Autodesk Inventor part; units mm, degrees
ref_plane "YZ Plane" through (0, 0, 0) normal (1, 0, 0) x (0, 1, 0)
ref_plane "XZ Plane" through (0, 0, 0) normal (0, 1, 0) x (-1, 0, 0)
ref_plane "XY Plane" through (0, 0, 0) normal (0, 0, 1) x (1, 0, 0)
sketch "Sketch1" plane through (0, 0, 0) normal (0, 0, 1) x (1, 0, 0)
  line L0 (-12.7, 12.7) -> (12.7, 12.7)
  line L1 (12.7, 12.7) -> (12.7, -12.7)
  line L2 (12.7, -12.7) -> (-12.7, -12.7)
  line L3 (-12.7, -12.7) -> (-12.7, 12.7)
  point P0 (0, 0)
  dimension "d0" = 25.4
  dimension "d1" = 25.4
  dimension "d2" = 12.7
  dimension "d3" = 12.7
extrude "Extrusion1" add sketch "Sketch1" along normal blind 50.8
sketch "Sketch2" plane through (0, 0, 50.8) normal (0, 0, 1) x (1, 0, 0)
  circle A0 centre (0, 0) radius 2.54
  line L0 (-4.5085, 4.5085) -> (4.5085, 4.5085)
  line L1 (-4.5085, -4.5085) -> (4.5085, -4.5085)
  line L2 (4.5085, 4.5085) -> (4.5085, -4.5085)
  line L3 (-4.5085, 4.5085) -> (-4.5085, -4.5085)
  line L4 (-3.0896, 4.5085) -> (-11.2811, 12.7)
  line L5 (-4.5085, 3.0537) -> (-12.7, 11.2452)
  line L6 (12.7, 12.7) -> (-12.7, 12.7)
  line L7 (-12.7, 12.7) -> (-12.7, 4.0005)
  line L8 (-10.668, 4.0005) -> (-10.668, 9.2132)
  line L9 (-9.2491, 10.668) -> (-3.3655, 10.668)
  line L10 (-12.7, 12.7) -> (-3.3655, 12.7)
  line L11 (-2.7305, 11.303) -> (-2.7305, 12.065)
  line L12 (-12.065, 3.3655) -> (-11.303, 3.3655)
  arc A1 (-12.7, 4.0005) -> (-12.065, 3.3655) centre (-12.065, 4.0005) ccw
  arc A2 (-11.303, 3.3655) -> (-10.668, 4.0005) centre (-11.303, 4.0005) ccw
  arc A3 (-3.3655, 10.668) -> (-2.7305, 11.303) centre (-3.3655, 11.303) ccw
  arc A4 (-2.7305, 12.065) -> (-3.3655, 12.7) centre (-3.3655, 12.065) ccw
  arc A5 (-3.3655, -11.303) -> (-4.0005, -10.668) centre (-4.0005, -11.303) ccw
  line L13 (-3.3655, -12.065) -> (-3.3655, -11.303)
  arc A6 (-4.0005, -12.7) -> (-3.3655, -12.065) centre (-4.0005, -12.065) ccw
  line L14 (-3.0537, -4.5085) -> (-11.2452, -12.7)
  line L15 (-10.668, -9.2491) -> (-10.668, -3.3655)
  line L16 (-4.5085, -3.0896) -> (-12.7, -11.2811)
  line L17 (-12.7, -12.7) -> (-12.7, -3.3655)
  arc A7 (-10.668, -3.3655) -> (-11.303, -2.7305) centre (-11.303, -3.3655) ccw
  line L18 (-11.303, -2.7305) -> (-12.065, -2.7305)
  arc A8 (-12.065, -2.7305) -> (-12.7, -3.3655) centre (-12.065, -3.3655) ccw
  line L19 (-4.0005, -10.668) -> (-9.2132, -10.668)
  line L20 (-12.7, -12.7) -> (-4.0005, -12.7)
  arc A9 (11.303, -3.3655) -> (10.668, -4.0005) centre (11.303, -4.0005) ccw
  line L21 (12.065, -3.3655) -> (11.303, -3.3655)
  arc A10 (12.7, -4.0005) -> (12.065, -3.3655) centre (12.065, -4.0005) ccw
  line L22 (4.5085, -3.0537) -> (12.7, -11.2452)
  line L23 (9.2491, -10.668) -> (3.3655, -10.668)
  line L24 (3.0896, -4.5085) -> (11.2811, -12.7)
  line L25 (12.7, -12.7) -> (3.3655, -12.7)
  arc A11 (3.3655, -10.668) -> (2.7305, -11.303) centre (3.3655, -11.303) ccw
  line L26 (2.7305, -11.303) -> (2.7305, -12.065)
  arc A12 (2.7305, -12.065) -> (3.3655, -12.7) centre (3.3655, -12.065) ccw
  line L27 (10.668, -4.0005) -> (10.668, -9.2132)
  line L28 (12.7, -12.7) -> (12.7, -4.0005)
  arc A13 (3.3655, 11.303) -> (4.0005, 10.668) centre (4.0005, 11.303) ccw
  line L29 (3.3655, 12.065) -> (3.3655, 11.303)
  arc A14 (4.0005, 12.7) -> (3.3655, 12.065) centre (4.0005, 12.065) ccw
  line L30 (3.0537, 4.5085) -> (11.2452, 12.7)
  line L31 (10.668, 9.2491) -> (10.668, 3.3655)
  line L32 (4.5085, 3.0896) -> (12.7, 11.2811)
  line L33 (12.7, 12.7) -> (12.7, 3.3655)
  arc A15 (10.668, 3.3655) -> (11.303, 2.7305) centre (11.303, 3.3655) ccw
  line L34 (11.303, 2.7305) -> (12.065, 2.7305)
  arc A16 (12.065, 2.7305) -> (12.7, 3.3655) centre (12.065, 3.3655) ccw
  line L35 (4.0005, 10.668) -> (9.2132, 10.668)
  line L36 (12.7, 12.7) -> (4.0005, 12.7)
  line L37 (-4.5085, 3.0537) -> (-4.5085, 4.5085)
  line L38 (-3.0896, 4.5085) -> (-4.5085, 4.5085)
  line L39 (-12.7, -12.7) -> (-4.0005, -12.7)
  line L40 (-4.0005, -10.668) -> (-9.2132, -10.668)
  line L41 (-10.668, -9.2491) -> (-10.668, -3.3655)
  line L42 (-12.7, -12.7) -> (-12.7, -3.3655)
  line L43 (-11.303, -2.7305) -> (-12.065, -2.7305)
  arc A17 (-10.668, -3.3655) -> (-11.303, -2.7305) centre (-11.303, -3.3655) ccw
  arc A18 (-12.065, -2.7305) -> (-12.7, -3.3655) centre (-12.065, -3.3655) ccw
  line L44 (-4.5085, -3.0896) -> (-4.5085, -4.5085)
  line L45 (-4.5085, -3.0896) -> (-12.7, -11.2811)
  line L46 (-3.0537, -4.5085) -> (-4.5085, -4.5085)
  line L47 (-3.0537, -4.5085) -> (-11.2452, -12.7)
  line L48 (-4.5085, -4.5085) -> (-4.5085, 4.5085)
  circle A19 centre (0, 0) radius 2.54
  line L49 (-4.5085, -4.5085) -> (4.5085, -4.5085)
  line L50 (-3.3655, -12.065) -> (-3.3655, -11.303)
  arc A20 (-4.0005, -12.7) -> (-3.3655, -12.065) centre (-4.0005, -12.065) ccw
  arc A21 (-3.3655, -11.303) -> (-4.0005, -10.668) centre (-4.0005, -11.303) ccw
  line L51 (12.7, -12.7) -> (12.7, -4.0005)
  line L52 (10.668, -4.0005) -> (10.668, -9.2132)
  line L53 (9.2491, -10.668) -> (3.3655, -10.668)
  line L54 (12.7, -12.7) -> (3.3655, -12.7)
  line L55 (2.7305, -11.303) -> (2.7305, -12.065)
  arc A22 (3.3655, -10.668) -> (2.7305, -11.303) centre (3.3655, -11.303) ccw
  arc A23 (2.7305, -12.065) -> (3.3655, -12.7) centre (3.3655, -12.065) ccw
  line L56 (3.0896, -4.5085) -> (4.5085, -4.5085)
  line L57 (3.0896, -4.5085) -> (11.2811, -12.7)
  line L58 (4.5085, -3.0537) -> (4.5085, -4.5085)
  line L59 (4.5085, -3.0537) -> (12.7, -11.2452)
  line L60 (4.5085, -4.5085) -> (-4.5085, -4.5085)
  circle A24 centre (0, 0) radius 2.54
  line L61 (4.5085, -4.5085) -> (4.5085, 4.5085)
  line L62 (12.065, -3.3655) -> (11.303, -3.3655)
  arc A25 (12.7, -4.0005) -> (12.065, -3.3655) centre (12.065, -4.0005) ccw
  arc A26 (11.303, -3.3655) -> (10.668, -4.0005) centre (11.303, -4.0005) ccw
  line L63 (12.7, 12.7) -> (4.0005, 12.7)
  line L64 (4.0005, 10.668) -> (9.2132, 10.668)
  line L65 (10.668, 9.2491) -> (10.668, 3.3655)
  line L66 (12.7, 12.7) -> (12.7, 3.3655)
  line L67 (11.303, 2.7305) -> (12.065, 2.7305)
  arc A27 (10.668, 3.3655) -> (11.303, 2.7305) centre (11.303, 3.3655) ccw
  arc A28 (12.065, 2.7305) -> (12.7, 3.3655) centre (12.065, 3.3655) ccw
  line L68 (4.5085, 3.0896) -> (4.5085, 4.5085)
  line L69 (4.5085, 3.0896) -> (12.7, 11.2811)
  line L70 (3.0537, 4.5085) -> (4.5085, 4.5085)
  line L71 (3.0537, 4.5085) -> (11.2452, 12.7)
  line L72 (4.5085, 4.5085) -> (4.5085, -4.5085)
  circle A29 centre (0, 0) radius 2.54
  line L73 (4.5085, 4.5085) -> (-4.5085, 4.5085)
  line L74 (3.3655, 12.065) -> (3.3655, 11.303)
  arc A30 (4.0005, 12.7) -> (3.3655, 12.065) centre (4.0005, 12.065) ccw
  arc A31 (3.3655, 11.303) -> (4.0005, 10.668) centre (4.0005, 11.303) ccw
  point P0 (-12.7, 3.3655)
  point P1 (-2.7305, 12.7)
  point P2 (-3.3655, -12.7)
  point P3 (-12.7, -2.7305)
  point P4 (12.7, -3.3655)
  point P5 (2.7305, -12.7)
  point P6 (3.3655, 12.7)
  point P7 (12.7, 2.7305)
  point P8 (-3.3655, -12.7)
  point P9 (-12.7, -2.7305)
  point P10 (12.7, -3.3655)
  point P11 (2.7305, -12.7)
  point P12 (3.3655, 12.7)
  point P13 (12.7, 2.7305)
  dimension "d6" = 5.08
  dimension "d7" = 9.017
  dimension "d8" = 4.5085
  dimension "d9" = 4.5085
  dimension "d10" = 4.5085
  dimension "d11" = 2.032
  dimension "d12" = 1.0033
  dimension "d13" = 135
  dimension "d17" = 9.3345
  dimension "d19" = 2.032
  dimension "d20" = 2.032
  dimension "d21" = 0.635
  dimension "d22" = 9.3345
  dimension "d25" = 360
  dimension "d29" = 360
extrude "Extrusion2" cut sketch "Sketch2" against normal up to surface (50.8 mm away) contours L3 L5 L7 L6 L4 L0 | L0 L2 L1 L3 | L30 L6 L33 L32 L2 L0 | L4 L6 A4 L11 A3 L9 | L3 L1 L14 L20 L17 L16 | L8 A2 L12 A1 L7 L5 | L35 A13 L29 A14 L6 L30 | L16 L17 A8 L18 A7 L15 | L22 L28 L25 L24 L1 L2 | L32 L33 A16 L34 A15 L31 | L19 A5 L13 A6 L20 L14 | L27 A9 L21 A10 L28 L22 | L24 L25 A12 L26 A11 L23 keep common part
equation "\"d22\" = d17"
properties part number "~2 in 80-20 extrusion"
Check sheet for the modelled part. Datum: model origin and axes. Units: mm. A direction names the side the tool comes from. Give positions to 0.01 mm unless a question says otherwise; leave off trailing zeros. Write each loop counter-clockwise with the first axis right and the second up, starting at its lowest first coordinate (ties: lowest second). Pieces come first, ordered by that corner, then holes. Notation, with made-up numbers: (19.5, -14) -> (74.5, -14) arc R23 ccw to (74.5, 2) -> close; hole circle Ø6 at (-2.75, 45.5). An arc over 180 degrees is marked (long way). Use CSV: the item, a comma, the result in double quotes. Start each with the question number.
Q1. Release check for a two-part mould opening along Y. For faces 3 (the flat face through (7, 10.668, 26)), 4 (the flat face through (0, 3, 0)), 5 (the flat face through (-8, 12.7, 25)) record: +Y half, -Y half, draft (parallel to the pull), parting line (faces both ways), or undercut.
Q2. Cross-section at C-C on y = -5.75. Enter the section's corners in (x, z).
Q3. Scan lines: line 1 along Y through (x, z) = (0, 38); line 2 along Y through (x, z) = (6.5, 10); line 3 along Y through (x, z) = (-5.5, 23). Record each from-to range of solid material in increasing order.
Q4. Cross-section at A-A on y = 0. Enter the section's corners in (x, z).
Q5. Tool access check on faces 1 (the flat face through (-6.09, -7.545, 25.756)), 2 (the flat face through (-8, -12.7, 25)). Record the directions out of +Z, -Z, +X, -X, +Y, -Y that give a thin tool (end or side, any length) a straight path to the whole face; none if there is none.
Q6. Depth check by flat-ended pin: P1, Ø1.5, axis at x = 4.5, y = -9.5, coming from the -Z side; P2, Ø4, axis at y = -3.5, z = 37, coming from the +X side; P3, Ø3, axis at x = 1, z = 30, coming from the -Y side; P4, Ø1.8, axis at y = 1, z = 25.5, coming from the +X side. Enter the tip coordinate at first touch or a pass-through.
Working result:
1,face 3,"undercut"
1,face 4,"draft"
1,face 5,"+Y half"
2,outline,"(-12.7, 0) -> (-10.67, 0) -> (-10.67, 50.8) -> (-12.7, 50.8) -> close; (-7.17, 0) -> (-4.3, 0) -> (-4.3, 50.8) -> (-7.17, 50.8) -> close; (4.33, 0) -> (7.2, 0) -> (7.2, 50.8) -> (4.33, 50.8) -> close; (10.67, 0) -> (12.7, 0) -> (12.7, 50.8) -> (10.67, 50.8) -> close"
3,line 1,"y = -4.51 to -2.54, 2.54 to 4.51"
3,line 2,"y = -12.7 to -10.67, -7.92 to -5.05, 5.08 to 7.95, 10.67 to 12.7"
3,line 3,"y = -12.7 to -10.67, -6.95 to -4.08, 4.05 to 6.92, 10.67 to 12.7"
4,outline,"(-4.51, 0) -> (-2.54, 0) -> (-2.54, 50.8) -> (-4.51, 50.8) -> close; (2.54, 0) -> (4.51, 0) -> (4.51, 50.8) -> (2.54, 50.8) -> close"
5,face 1,"+Z, -Z"
5,face 2,"+Z, -Z, +X, -X, -Y"
6,P1,"passes through"
6,P2,"stops at x = 12.7"
6,P3,"stops at y = -4.51"
6,P4,"stops at x = 4.51"
